Check sheet for the modelled part. Datum: model origin and axes. Units: mm. Face numbers are marked on the shaded views. A direction names the side the tool comes from. Give positions to 0.01 mm unless a question says otherwise; leave off trailing zeros. Order: outer loops, then holes, each group sorted by start corner. A loop starts at its lowest first (then second) coordinate and runs counter-clockwise, first axis right, second up.
Autodesk Inventor part; units mm, degrees
ref_plane "YZ Plane" through (0, 0, 0) normal (1, 0, 0) x (0, 1, 0)
ref_plane "XZ Plane" through (0, 0, 0) normal (0, 1, 0) x (-1, 0, 0)
ref_plane "XY Plane" through (0, 0, 0) normal (0, 0, 1) x (1, 0, 0)
sketch "Sketch1" plane through (0, 0, 0) normal (0, 0, 1) x (1, 0, 0)
  line L0 (0, 0) -> (0, 19)
  line L1 (0, 19) -> (34.5, 19)
  line L2 (34.5, 19) -> (34.5, 10)
  line L3 (34.5, 10) -> (39.5, 10)
  line L4 (39.5, 10) -> (39.5, 3)
  line L5 (39.5, 3) -> (51.5, 3)
  line L6 (51.5, 3) -> (51.5, 0)
  line L7 (51.5, 0) -> (0, 0)
  dimension "d0" = 19
  dimension "d1" = 34.5
  dimension "d2" = 5
  dimension "d3" = 10
  dimension "d4" = 12
  dimension "d5" = 3
revolve "Revolution1" add sketch "Sketch1" angle 360 about axis through (51.5, 0, 0) along (-1, 0, 0)
sketch "Sketch2" plane through (51.5, 0, 0) normal (1, 0, 0) x (0, 0, -1)
  circle A0 centre (0, 0) radius 3
  circle A1 centre (0, 0) radius 3
  line L0 (-1.6583, 2.5) -> (1.6583, 2.5)
  point P0 (0, 0)
  point P1 (-1.6583, 2.5)
  point P2 (1.6583, 2.5)
  dimension "d7" = 2.5
extrude "Extrusion1" cut sketch "Sketch2" against normal blind 10 contours L0 A0 picked at (-0.1169, 2.6598)
sketch "Sketch3" plane through (34.5, 0, 0) normal (1, 0, 0) x (0, 0, -1)
  circle A0 centre (0, 15) radius 1.25
  circle A1 centre (4.7883, 13.1557) radius 1.25
  circle A2 centre (0, 0) radius 3
  circle A3 centre (0, 0) radius 14 construction
  circle A4 centre (0, 0) radius 15 construction
  circle A5 centre (0, 0) radius 19
  line L0 (0, 0) -> (0, 15) construction
  line L1 (1.6583, 2.5) -> (-1.6583, 2.5)
  line L2 (0, 0) -> (4.7883, 13.1557) construction
  circle A6 centre (-13.7873, -2.4311) radius 1.25
  circle A7 centre (-12.9904, -7.5) radius 1.25
  circle A8 centre (8.999, -10.7246) radius 1.25
  circle A9 centre (12.9904, -7.5) radius 1.25
  dimension "d21" = 28
  dimension "d22" = 30
  dimension "d10" = 4
  dimension "d11" = 5
  dimension "d12" = 2.5
  dimension "d13" = 2.5
  dimension "d14" = 20
  dimension "d17" = 360
extrude "Extrusion2" cut sketch "Sketch3" against normal blind 10 contours A0 | A1 | A2 L1 | L1 A2 | A6 | A7 | A8 | A9
properties part number "TestEncoder"
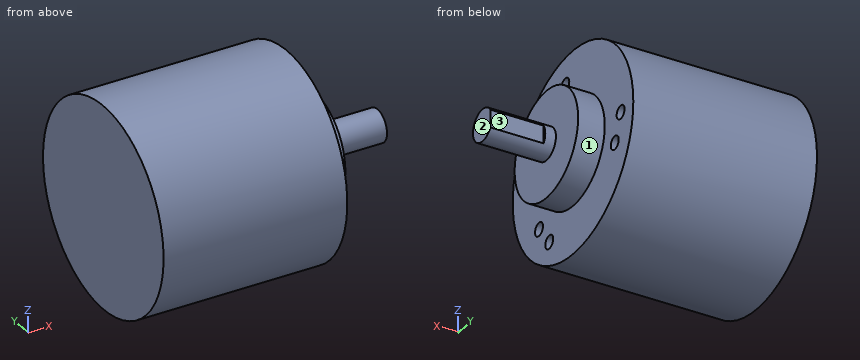
(1) Thickness scan on L1, parallel to Y at x = 30.25, z = 0; L2, parallel to Y at x = 33, z = 0.5; L3, parallel to Z at x = 30, y = -7. Record the ranges inside material, lowest first.
(2) Tool access check on the marked faces 1, 2 and 3. Record the directions out of +Z, -Z, +X, -X, +Y, -Y that give a thin tool (end or side, any length) a straight path to the whole face; none if there is none.
(3) Sectioned sample at A-A (z = 0). Enter the section's corners in (x, y).
(4) Sectioned sample at D-D (z = -13.5). Enter the section's corners in (x, y).
(5) Sectioned sample at B-B (y = 0). Enter the section's corners in (x, z).
(6) Go/stop test with flat-tipped pins: P1, Ø4, axis at y = 0, z = 4, coming from the +X side; P2, Ø0.8, axis at y = 12.5, z = -5, coming from the +X side; P3, Ø5, axis at x = 10, z = -14.5, coming from the -Y side; P4, Ø1.5, axis at x = 36, z = 8, coming from the +Y side. Record where each tip stops, or that it passes through.
(7) Sectioned sample at C-C (x = 30). Enter the section's corners in (y, z), plus the area to 3 significant figures.
Values follow:
1. L1: y = -19 to -3, 3 to 13.75, 16.25 to 19
1. L2: y = -18.99 to -2.96, 2.96 to 13.85, 16.15 to 18.99
1. L3: z = -17.66 to -14.14, -11.84 to 11.84, 14.14 to 17.66
2. face 1: +X
2. face 2: +Z, -Z, +X, +Y, -Y
2. face 3: +Z, -Z, +X, +Y
3. outline: (0, -19) - (34.5, -19) - (34.5, -10) - (39.5, -10) - (39.5, -3) - (51.5, -3) - (51.5, 2.5) - (41.5, 2.5) - (41.5, 3) - (39.5, 3) - (39.5, 10) - (34.5, 10) - (34.5, 13.75) - (24.5, 13.75) - (24.5, 16.25) - (34.5, 16.25) - (34.5, 19) - (0, 19) - close; hole (24.5, -3) - (34.5, -3) - (34.5, 3) - (24.5, 3) - close
4. outline: (0, -13.37) - (34.5, -13.37) - (34.5, -8.64) - (24.5, -8.64) - (24.5, -6.36) - (34.5, -6.36) - (34.5, 13.37) - (0, 13.37) - close
5. outline: (0, -19) - (34.5, -19) - (34.5, -10) - (39.5, -10) - (39.5, -3) - (51.5, -3) - (51.5, 3) - (39.5, 3) - (39.5, 10) - (34.5, 10) - (34.5, 19) - (0, 19) - close; hole (24.5, -3) - (34.5, -3) - (34.5, 3) - (24.5, 3) - close
6. P1: stops at x = 51.5
6. P2: stops at x = 24.5
6. P3: stops at y = -14.73
6. P4: stops at y = 6.89
7. outline: circle Ø38 at (0, 0); hole circle Ø2.5 at (-10.72, -9); hole circle Ø2.5 at (-7.5, -12.99); hole circle Ø2.5 at (-7.5, 12.99); hole circle Ø2.5 at (-2.43, 13.79); hole circle Ø6 at (0, 0); hole circle Ø2.5 at (13.16, -4.79); hole circle Ø2.5 at (15, 0)
7. area: 1,080 mm2
